Here's how the part is built. I have some questions about the finished solid (model axes, mm). A direction names the side the tool comes from. Round coordinates to 2 decimals unless told otherwise and drop trailing zeros. Write each loop counter-clockwise with the first axis right and the second up, starting at its lowest first coordinate (ties: lowest second). Pieces come first, ordered by that corner, then holes. Notation, with made-up numbers: M -3.5,57 L 14.5,57 A18 cw 14.5,68 Z; hole C 22,-17 d4. An arc over 180 degrees is marked long. Use a Markdown table: item, result. Add a question column.
```python
from build123d import *

# Parameters (mm, degrees)
BOSS_EXTRUDE1_DEPTH = 4.75
CUT_EXTRUDE1_REACH  = 11.471
CUT_EXTRUDE2_DEPTH  = 0.85


with BuildPart() as part:
    # Sketch1 → Boss-Extrude1 (new body)
    with BuildSketch(Plane(origin=(0, 0, 0), x_dir=(0, 0, -1), z_dir=(1, 0, 0))):
        Polygon((0, 0.15), (0, 7.05), (-0.241393443, 8.15), (-0.647131148, 8.15), (-0.85, 7.05), (-0.85, 0.15), align=None)
    extrude(amount=BOSS_EXTRUDE1_DEPTH)

    # Cut-Extrude1: up to this face of the body (flat: up to its plane)
    cut_extrude1_end = Plane(part.part.faces().sort_by_distance((2.375, 3.6, 0))[0])
    # Sketch4 → Cut-Extrude1 (cut, up to the picked face)
    with BuildSketch(Plane.XY.offset(0.85), mode=Mode.PRIVATE) as cut_extrude1_sk1:
        Polygon((0, 6.9), (1.25, 8.15), (0, 8.15), align=None)
    cut_extrude1_tool1 = split(extrude(cut_extrude1_sk1.sketch, amount=-CUT_EXTRUDE1_REACH, mode=Mode.PRIVATE), bisect_by=cut_extrude1_end, keep=Keep.BOTH, mode=Mode.PRIVATE)
    # Sketch4 → Cut-Extrude1 (cut, up to the picked face)
    with BuildSketch(Plane.XY.offset(0.85), mode=Mode.PRIVATE) as cut_extrude1_sk2:
        Polygon((3.5, 8.15), (4.75, 6.9), (4.75, 8.15), align=None)
    cut_extrude1_tool2 = split(extrude(cut_extrude1_sk2.sketch, amount=-CUT_EXTRUDE1_REACH, mode=Mode.PRIVATE), bisect_by=cut_extrude1_end, keep=Keep.BOTH, mode=Mode.PRIVATE)
    add(cut_extrude1_tool1.solids().sort_by(Axis((0.416667, 7.733333, 0.85), (0, 0, -1)))[0], mode=Mode.SUBTRACT)
    add(cut_extrude1_tool2.solids().sort_by(Axis((4.333333, 7.733333, 0.85), (0, 0, -1)))[0], mode=Mode.SUBTRACT)

    # Sketch5 → Cut-Extrude2 (cut)
    with BuildSketch(Plane.XY.offset(0.85)):
        with BuildLine():
            Line((1.913461538, 5.842307692), (1.451923077, 4.734615385))
            ThreePointArc((1.451923077, 4.734615385), (2.37510742, 3.350000006), (3.297994271, 4.734813689))
            Line((3.297994271, 4.734813689), (2.842436975, 5.827489929))
            ThreePointArc((2.842436975, 5.827489929), (2.382974312, 6.149936406), (1.913461538, 5.842307692))
        make_face()
    extrude(amount=-CUT_EXTRUDE2_DEPTH, mode=Mode.SUBTRACT)


solid = part.part
```
Item 1: On a 3-axis mill with a long thin cutter (end or side, diameter ignored), from which of +Z, -Z, +X, -X, +Y, -Y can I reach the whole of each face in a straight line? I mean faces 1 (the face through (4.75, 3.6, 0.4)), 2 (the face through (3.073, 5.274, 0.431)). Say none if no direction works.
Item 2: I need wall thicknesses on probe 1 along X at (y, z) = (4.35, 0.4) (3 decimals); probe 2 along X at (y, z) = (3.5, 0.75); probe 3 along Y at (x, z) = (2.85, 0.55). Which ranges of each line are inside material? Lowest first, please. Write a range as from..to.
Item 3: Imagine slicing it at A-A on y = 4.35. List the corners of the cut face in (x, z) for me (3 decimals).
Item 4: Imagine slicing it at B-B on x = 1.75. List the corners of the cut face in (y, z) for me, plus the area to 3 significant figures.
Item 5: Imagine slicing it at C-C on z = 0.4. List the corners of the cut face in (x, y) for me (3 decimals).
Item 6: If we mould it in two halves opening along Y, with no side actions, what happens to faces 3 (the face through (2.35, 3.35, 0.43)), 4 (the face through (2, 3, 0)), 5 (the face through (0.5, 7.4, 0.4))? For each: +Y half, -Y half, draft (parallel to the pull), parting line (faces both ways), or undercut.
Item 7: Imagine slicing it at D-D on y = 3.5. List the corners of the cut face in (x, z) for me, plus the area to 3 significant figures.
The answers:
| question | item | result |
|---|---|---|
| 1 | face 1 | +Z, -Z, +X, +Y, -Y |
| 1 | face 2 | +Z, -Z |
| 2 | probe 1 | 0..1.375, 3.375..4.75 |
| 2 | probe 2 | 0..1.85, 2.9..4.75 |
| 2 | probe 3 | 0.15..3.47, 5.81..8.15 |
| 3 | outline | M 0,0 L 1.375,0 L 1.375,0.85 L 0,0.85 Z; M 3.375,0 L 4.75,0 L 4.75,0.85 L 3.375,0.85 Z |
| 4 | outline | M 0.15,0 L 3.57,0 L 3.57,0.85 L 0.15,0.85 Z; M 5.45,0 L 7.05,0 L 8.15,0.24 L 8.15,0.65 L 7.05,0.85 L 5.45,0.85 Z |
| 4 | area | 4.96 mm² |
| 5 | outline | M 0,0.15 L 4.75,0.15 L 4.75,6.9 L 3.5,8.15 L 1.25,8.15 L 0,6.9 Z; hole M 1.452,4.735 A1 ccw long 3.298,4.735 L 2.842,5.827 A0.5 ccw 1.913,5.842 Z |
| 6 | face 3 | undercut |
| 6 | face 4 | draft |
| 6 | face 5 | +Y half |
| 7 | outline | M 0,0 L 1.85,0 L 1.85,0.85 L 0,0.85 Z; M 2.9,0 L 4.75,0 L 4.75,0.85 L 2.9,0.85 Z |
| 7 | area | 3.14 mm² |
